from build123d import *

# Parameters (mm, degrees)
BOSS_EXTRUDE1_DEPTH = 4
BOSS_EXTRUDE3_DEPTH = 2
BOSS_EXTRUDE4_DEPTH = 4


with BuildPart() as part:
    # Sketch2 → Boss-Extrude1 (new body)
    with BuildSketch(Plane(origin=(0, 0, 0), x_dir=(1, 0, 0), z_dir=(0, 1, 0))):
        with BuildLine():
            Line((0.12816248, 0), (0.19140299, 0))
            Line((0.19140299, 0), (0.580035518, 0))
            Line((0.580035518, 0), (8, 0))
            Line((8, 0), (8.04118409, 0))
            ThreePointArc((8.04118409, 0), (13.15, 4.5), (18.25881591, 0))
            Line((18.25881591, 0), (18.3, 0))
            Line((18.3, 0), (26.3, 0))
            Line((26.3, 0), (27.90423081, 0))
            Line((27.90423081, 0), (42.8, 0))
            Line((42.8, 0), (52.528764428, 8.163402643))
            Line((52.528764428, 8.163402643), (42.8, 8.163402643))
            Line((42.8, 8.163402643), (42.8, 1.5))
            Line((42.8, 1.5), (26.3, 1.5))
            Line((26.3, 1.5), (26.3, 13.7))
            Line((26.3, 13.7), (-7.372368399, 13.7))
            Line((-7.372368399, 13.7), (-7.372368399, 5.162187927))
            Line((-7.372368399, 5.162187927), (0, 0))
            Line((0, 0), (0.12816248, 0))
        make_face()
        with BuildLine():
            ThreePointArc((18.25881591, 0), (13.15, 4.5), (8.04118409, 0))
            Line((8.04118409, 0), (8.088379706, 0))
            ThreePointArc((8.088379706, 0), (8.155534558, 0.306111042), (8.24118409, 0.607570661))
            ThreePointArc((8.24118409, 0.607570661), (10.108535624, 3.205958909), (13.15, 4.2))
            ThreePointArc((13.15, 4.2), (16.191464376, 3.205958909), (18.05881591, 0.607570661))
            ThreePointArc((18.05881591, 0.607570661), (18.144465442, 0.306111042), (18.211620294, 0))
            Line((18.211620294, 0), (18.25881591, 0))
        make_face()
        with BuildLine():
            ThreePointArc((13.15, 4.2), (10.108535624, 3.205958909), (8.24118409, 0.607570661))
            Line((8.24118409, 0.607570661), (8.24118409, 0))
            Line((8.24118409, 0), (13.15, 0))
            Line((13.15, 0), (13.15, 4.2))
        make_face()
        with BuildLine():
            ThreePointArc((18.05881591, 0.607570661), (16.191464376, 3.205958909), (13.15, 4.2))
            Line((13.15, 4.2), (13.15, 0))
            Line((13.15, 0), (18.05881591, 0))
            Line((18.05881591, 0), (18.05881591, 0.607570661))
        make_face()
        Polygon((13.15, 0), (8.24118409, 0), (8.24118409, -0.3), (18.05881591, -0.3), (18.05881591, 0), align=None)
        with BuildLine():
            ThreePointArc((8.24118409, 0.607570661), (8.155534558, 0.306111042), (8.088379706, 0))
            ThreePointArc((8.088379706, 0), (8.062570085, -0.14965204), (8.04118409, -0.3))
            Line((8.04118409, -0.3), (8.24118409, -0.3))
            Line((8.24118409, -0.3), (8.24118409, 0))
            Line((8.24118409, 0), (8.24118409, 0.607570661))
        make_face()
        with BuildLine():
            ThreePointArc((18.25881591, -0.3), (18.237429915, -0.14965204), (18.211620294, 0))
            ThreePointArc((18.211620294, 0), (18.144465442, 0.306111042), (18.05881591, 0.607570661))
            Line((18.05881591, 0.607570661), (18.05881591, 0))
            Line((18.05881591, 0), (18.05881591, -0.3))
            Line((18.05881591, -0.3), (18.25881591, -0.3))
        make_face()
        with BuildLine():
            Line((18.3, 0), (18.25881591, 0))
            Line((18.25881591, 0), (18.211620294, 0))
            ThreePointArc((18.211620294, 0), (18.237429915, -0.14965204), (18.25881591, -0.3))
            Line((18.25881591, -0.3), (42.8, -0.3))
            Line((42.8, -0.3), (42.992836283, -0.229813333))
            Line((42.992836283, -0.229813333), (43.639486744, 0.312790831))
            Line((43.639486744, 0.312790831), (52.721600711, 7.93358931))
            Line((52.721600711, 7.93358931), (52.528764428, 8.163402643))
            Line((52.528764428, 8.163402643), (42.8, 0))
            Line((42.8, 0), (27.90423081, 0))
            Line((27.90423081, 0), (26.3, 0))
            Line((26.3, 0), (18.3, 0))
        make_face()
        Polygon((-0.094589637, -0.3), (-7.54444133, 4.916442314), (-9.666674144, 1.88557975), (-1.261195156, -4), (0, -4), (42.8, -4), (45.371150439, -3.064177772), (55.099914866, 5.099224871), (52.721600711, 7.93358931), (43.639486744, 0.312790831), (42.992836283, -0.229813333), (42.8, -0.3), (18.25881591, -0.3), (18.05881591, -0.3), (8.24118409, -0.3), (8.04118409, -0.3), (0, -0.3), align=None)
        with BuildLine():
            Line((0.580035518, 0), (0.19140299, 0))
            Line((0.19140299, 0), (0.12816248, 0))
            Line((0.12816248, 0), (0, 0))
            Line((0, 0), (-7.372368399, 5.162187927))
            Line((-7.372368399, 5.162187927), (-7.54444133, 4.916442314))
            Line((-7.54444133, 4.916442314), (-0.094589637, -0.3))
            Line((-0.094589637, -0.3), (0, -0.3))
            Line((0, -0.3), (8.04118409, -0.3))
            ThreePointArc((8.04118409, -0.3), (8.062570085, -0.14965204), (8.088379706, 0))
            Line((8.088379706, 0), (8.04118409, 0))
            Line((8.04118409, 0), (8, 0))
            Line((8, 0), (0.580035518, 0))
        make_face()
    extrude(amount=BOSS_EXTRUDE1_DEPTH)

    # Sketch2_4 → Boss-Extrude3 (add)
    with BuildSketch(Plane(origin=(0, 0, 0), x_dir=(1, 0, 0), z_dir=(0, 1, 0))):
        Polygon((-0.094589637, -0.3), (-7.54444133, 4.916442314), (-9.666674144, 1.88557975), (-1.261195156, -4), (0, -4), (42.8, -4), (45.371150439, -3.064177772), (55.099914866, 5.099224871), (52.721600711, 7.93358931), (43.639486744, 0.312790831), (42.992836283, -0.229813333), (42.8, -0.3), (18.25881591, -0.3), (18.05881591, -0.3), (8.24118409, -0.3), (8.04118409, -0.3), (0, -0.3), align=None)
        with BuildLine():
            ThreePointArc((18.05881591, 0.607570661), (16.191464376, 3.205958909), (13.15, 4.2))
            Line((13.15, 4.2), (13.15, 0))
            Line((13.15, 0), (18.05881591, 0))
            Line((18.05881591, 0), (18.05881591, 0.607570661))
        make_face()
        with BuildLine():
            ThreePointArc((13.15, 4.2), (10.108535624, 3.205958909), (8.24118409, 0.607570661))
            Line((8.24118409, 0.607570661), (8.24118409, 0))
            Line((8.24118409, 0), (13.15, 0))
            Line((13.15, 0), (13.15, 4.2))
        make_face()
        Polygon((13.15, 0), (8.24118409, 0), (8.24118409, -0.3), (18.05881591, -0.3), (18.05881591, 0), align=None)
    extrude(amount=-BOSS_EXTRUDE3_DEPTH)

    # Sketch3 → Boss-Extrude4 (add)
    with BuildSketch(Plane(origin=(0, -2, 0), x_dir=(-1, 0, 0), z_dir=(0, -1, 0))):
        with BuildLine():
            Line((-18.25881591, 5.162187927), (-18.25881591, 0))
            ThreePointArc((-18.25881591, 0), (-13.15, 4.5), (-8.04118409, 0))
            Line((-8.04118409, 0), (-8, 0))
            Line((-8, 0), (-0.580035518, 0))
            Line((-0.580035518, 0), (-0.19140299, 0))
            Line((-0.19140299, 0), (-0.12816248, 0))
            Line((-0.12816248, 0), (0, 0))
            Line((0, 0), (7.372368399, 5.162187927))
            Line((7.372368399, 5.162187927), (-18.25881591, 5.162187927))
        make_face()
        Polygon((-52.528764428, 10.163402643), (-52.528764428, 8.163402643), (-44.028764428, 1.031055778), (-44.028764428, 8.163402643), (-44.028764428, 10.163402643), align=None)
        with BuildLine():
            Line((-44.028764428, 1.031055778), (-52.528764428, 8.163402643))
            Line((-52.528764428, 8.163402643), (-52.721600711, 7.93358931))
            Line((-52.721600711, 7.93358931), (-43.639486744, 0.312790831))
            Line((-43.639486744, 0.312790831), (-42.992836283, -0.229813333))
            Line((-42.992836283, -0.229813333), (-42.8, -0.3))
            Line((-42.8, -0.3), (-18.25881591, -0.3))
            ThreePointArc((-18.25881591, -0.3), (-18.237429915, -0.14965204), (-18.211620294, 0))
            Line((-18.211620294, 0), (-18.25881591, 0))
            Line((-18.25881591, 0), (-18.3, 0))
            Line((-18.3, 0), (-26.3, 0))
            Line((-26.3, 0), (-27.90423081, 0))
            Line((-27.90423081, 0), (-42.8, 0))
            Line((-42.8, 0), (-44.028764428, 1.031055778))
        make_face()
        Polygon((-43.639486744, 0.312790831), (-52.721600711, 7.93358931), (-55.099914866, 5.099224871), (-45.371150439, -3.064177772), (-42.8, -4), (0, -4), (1.261195156, -4), (9.666674144, 1.88557975), (7.54444133, 4.916442314), (0.094589637, -0.3), (0, -0.3), (-8.04118409, -0.3), (-8.24118409, -0.3), (-18.05881591, -0.3), (-18.25881591, -0.3), (-42.8, -0.3), (-42.992836283, -0.229813333), align=None)
        with BuildLine():
            Line((-13.15, 4.2), (-13.15, 0))
            Line((-13.15, 0), (-8.24118409, 0))
            Line((-8.24118409, 0), (-8.24118409, 0.607570661))
            ThreePointArc((-8.24118409, 0.607570661), (-10.108535624, 3.205958909), (-13.15, 4.2))
        make_face()
        with BuildLine():
            Line((-18.05881591, 0.607570661), (-18.05881591, 0))
            Line((-18.05881591, 0), (-13.15, 0))
            Line((-13.15, 0), (-13.15, 4.2))
            ThreePointArc((-13.15, 4.2), (-16.191464376, 3.205958909), (-18.05881591, 0.607570661))
        make_face()
        with BuildLine():
            Line((-8.24118409, 0), (-8.24118409, -0.3))
            Line((-8.24118409, -0.3), (-8.04118409, -0.3))
            ThreePointArc((-8.04118409, -0.3), (-8.062570085, -0.14965204), (-8.088379706, 0))
            ThreePointArc((-8.088379706, 0), (-8.155534558, 0.306111042), (-8.24118409, 0.607570661))
            Line((-8.24118409, 0.607570661), (-8.24118409, 0))
        make_face()
        Polygon((-18.05881591, 0), (-18.05881591, -0.3), (-8.24118409, -0.3), (-8.24118409, 0), (-13.15, 0), align=None)
        with BuildLine():
            Line((-8, 0), (-8.04118409, 0))
            Line((-8.04118409, 0), (-8.088379706, 0))
            ThreePointArc((-8.088379706, 0), (-8.062570085, -0.14965204), (-8.04118409, -0.3))
            Line((-8.04118409, -0.3), (0, -0.3))
            Line((0, -0.3), (0.094589637, -0.3))
            Line((0.094589637, -0.3), (7.54444133, 4.916442314))
            Line((7.54444133, 4.916442314), (7.372368399, 5.162187927))
            Line((7.372368399, 5.162187927), (0, 0))
            Line((0, 0), (-0.12816248, 0))
            Line((-0.12816248, 0), (-0.19140299, 0))
            Line((-0.19140299, 0), (-0.580035518, 0))
            Line((-0.580035518, 0), (-8, 0))
        make_face()
        with BuildLine():
            Line((-18.25881591, 0), (-18.211620294, 0))
            ThreePointArc((-18.211620294, 0), (-18.144465442, 0.306111042), (-18.05881591, 0.607570661))
            ThreePointArc((-18.05881591, 0.607570661), (-16.191464376, 3.205958909), (-13.15, 4.2))
            ThreePointArc((-13.15, 4.2), (-10.108535624, 3.205958909), (-8.24118409, 0.607570661))
            ThreePointArc((-8.24118409, 0.607570661), (-8.155534558, 0.306111042), (-8.088379706, 0))
            Line((-8.088379706, 0), (-8.04118409, 0))
            ThreePointArc((-8.04118409, 0), (-13.15, 4.5), (-18.25881591, 0))
        make_face()
        with BuildLine():
            ThreePointArc((-18.211620294, 0), (-18.237429915, -0.14965204), (-18.25881591, -0.3))
            Line((-18.25881591, -0.3), (-18.05881591, -0.3))
            Line((-18.05881591, -0.3), (-18.05881591, 0))
            Line((-18.05881591, 0), (-18.05881591, 0.607570661))
            ThreePointArc((-18.05881591, 0.607570661), (-18.144465442, 0.306111042), (-18.211620294, 0))
        make_face()
    extrude(amount=BOSS_EXTRUDE4_DEPTH)


solid = part.part
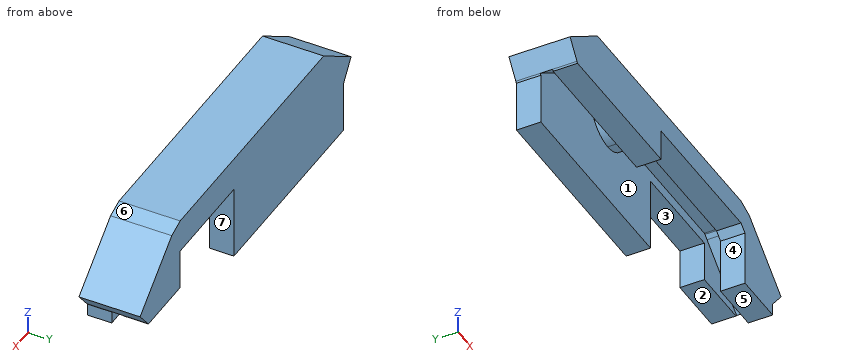
Check sheet for the modelled part. Datum: model origin and axes. Units: mm. Face numbers are marked on the shaded views. A direction names the side the tool comes from. Give positions to 0.01 mm unless a question says otherwise; leave off trailing zeros. Loops run counter-clockwise (first coordinate to the right, second up) from the corner with the lowest first, then second, coordinate; pieces in that order, holes last. Notation, with made-up numbers: M 31,-27 L 86,-27 A19 ccw 86,2 Z; hole C -27.5,-9.5 d3. An arc over 180 degrees is marked long. Return JSON: item names as keys, results as strings. Group by question number.
1. Cross-section at C-C on z = -6. Record the boundary of the cut face in (x, y), plus the area to 3 significant figures.
2. Thickness scan on L1, parallel to Y at x = 49, z = -5; L2, parallel to X at y = -0.5, z = -2.25; L3, parallel to Z at x = 24.5, y = -2.5. Record the ranges inside material, lowest first.
3. Cross-section at D-D on y = 2.75. Record the boundary of the cut face in (x, z), plus the area to 3 significant figures.
4. Cross-section at A-A on x = 21. Record the boundary of the cut face in (y, z), plus the area to 3 significant figures.
5. Cross-section at B-B on y = -3.5. Record the boundary of the cut face in (x, z).
6. Mould release check, pull along X, two halves, no side actions. Record for the marked faces 5, 6 and 7: released by +X, released by -X, zero draft, split by the parting line, or undercut.
7. Go/stop test with flat-tipped pins: pin 1 (1 mm diameter, centred on x = 20, z = -8.5, fed in from -Y); pin 2 (3 mm diameter, centred on y = 1, z = -8.5, fed in from -X); pin 3 (0.7 mm diameter, centred on y = -1, z = 0, fed in from -X). Record where each tip stops, or that it passes through.
8. Tool access check on the marked faces 1, 2, 3 and 4. Record the directions out of +Z, -Z, +X, -X, +Y, -Y that give a thin tool (end or side, any length) a straight path to the whole face; none if there is none.
Return value:
{
 "1": {"outline": "M -7.37,0 L 26.3,0 L 26.3,4 L -7.37,4 Z; M 42.8,0 L 50.42,0 L 50.42,-2 L 44.03,-2 L 44.03,-6 L 54.34,-6 L 54.34,4 L 42.8,4 Z", "area": "230 mm^2"},
 "2": {"L1": "-6 to -2, 0 to 4", "L2": "-9.41 to -3.74, 9.11 to 17.19, 45.95 to 51.7", "L3": "0 to 4"},
 "3": {"outline": "M -9.67,-1.89 L -7.37,-5.16 L -7.37,-13.7 L 26.3,-13.7 L 26.3,-1.5 L 42.8,-1.5 L 42.8,-8.16 L 52.53,-8.16 L 55.1,-5.1 L 45.37,3.06 L 42.8,4 L -1.26,4 Z", "area": "775 mm^2"},
 "4": {"outline": "M -6,0 L -2,0 L -2,0.3 L 0,0.3 L 0,-13.7 L 4,-13.7 L 4,4 L -6,4 Z", "area": "94.2 mm^2"},
 "5": {"outline": "M -9.67,-1.89 L -7.37,-5.16 L 18.26,-5.16 L 18.26,0 L 42.8,0 L 44.03,-1.03 L 44.03,-10.16 L 52.53,-10.16 L 52.53,-8.16 L 55.1,-5.1 L 45.37,3.06 L 42.8,4 L -1.26,4 Z"},
 "6": {"face 5": "zero draft", "face 6": "released by +X", "face 7": "undercut"},
 "7": {"pin 1": "y = 0", "pin 2": "x = -7.37", "pin 3": "x = -7.47"},
 "8": {"face 1": "-Z", "face 2": "-Z, +X, +Y", "face 3": "-Z, +Y, -Y", "face 4": "-Z, -Y"}
}
